For this review, take the finished solid that the model builds, in its own axes (mm). Give positions to 0.01 mm unless a question says otherwise; leave off trailing zeros. Write each loop counter-clockwise with the first axis right and the second up, starting at its lowest first coordinate (ties: lowest second). Pieces come first, ordered by that corner, then holes.
Q1. We need section A-A (y = 63.5). Write out the cut boundary in (x, z).
Q2. For line 1 (Y direction, x = 111.5, z = 4.75); line 2 (Y direction, x = 125, z = 1.2); line 3 (X direction, y = 19.5, z = 1.9), list the stretches that pass through material, from the lowest coordinate up.
Q3. Insertion check: P1, Ø1.8, axis at x = 105.72, y = -7.19, coming from the -Z side; P2, Ø3.5, axis at x = 125.72, y = 83.81, coming from the +Z side. Each pin has a flat end and moves straight along its axis. Give the tip position at first contact, or say it passes through.
Q4. We need section C-C (z = 3.15). Give the number of separate pieces and of enclosed holes in the cut face, then the cut area to 3 significant figures.
Q5. We need section B-B (x = 92.5). Write out the cut boundary in (y, z).
Q6. We need section D-D (x = 99.5). Write out the cut boundary in (y, z), then the cut area to 3 significant figures.
Autodesk Fusion 360 part; units mm, degrees
sketch "Schizzo5" plane through (0, 0, 0) normal (0, 0, 1) x (1, 0, 0)
  line L0 (80.7173, 86.3147) -> (80.7173, -9.6853)
  circle A0 centre (85.7173, -7.1853) radius 1.5
  circle A1 centre (105.7173, 38.3147) radius 25 construction
  arc A2 (125.5163, 58.1137) -> (105.7173, 66.3147) centre (105.7173, 38.3147) ccw
  circle A3 centre (121.787, 57.4658) radius 3
  circle A4 centre (89.6476, 57.4658) radius 3
  arc A5 (105.7173, 66.3147) -> (85.9183, 58.1137) centre (105.7173, 38.3147) ccw
  circle A6 centre (125.7173, 83.8147) radius 3
  arc A7 (105.7173, 10.3147) -> (125.5163, 18.5157) centre (105.7173, 38.3147) ccw
  line L1 (80.7173, 38.3147) -> (130.7173, 38.3147) construction
  circle A8 centre (105.7173, 83.8147) radius 1.5
  circle A9 centre (85.7173, 83.8147) radius 3
  line L2 (105.7173, 38.3147) -> (121.787, 19.1636) construction
  arc A10 (105.7173, 66.3147) -> (85.9183, 58.1137) centre (105.7173, 38.3147) ccw
  circle A11 centre (85.7173, 83.8147) radius 1.5
  line L3 (130.7173, 86.3147) -> (80.7173, 86.3147)
  arc A12 (125.5163, 58.1137) -> (105.7173, 66.3147) centre (105.7173, 38.3147) ccw
  circle A13 centre (125.7173, 83.8147) radius 1.5
  line L4 (105.7173, 38.3147) -> (89.6274, 54.4047) construction
  circle A14 centre (105.7173, 83.8147) radius 3
  arc A15 (105.7173, 10.3147) -> (125.5163, 18.5157) centre (105.7173, 38.3147) ccw
  line L5 (105.7173, 38.3147) -> (105.7173, 13.3147) construction
  circle A16 centre (105.7173, 38.3147) radius 4.1
  circle A17 centre (105.7173, -7.1853) radius 1.5
  circle A18 centre (89.6476, 19.1636) radius 3
  line L6 (130.7173, -9.6853) -> (130.7173, 86.3147)
  arc A19 (85.9183, 18.5157) -> (105.7173, 10.3147) centre (105.7173, 38.3147) ccw
  line L7 (85.7173, 86.3147) -> (85.7173, -9.6853) construction
  arc A20 (105.7173, 13.3147) -> (121.787, 19.1636) centre (105.7173, 38.3147) ccw
  circle A21 centre (121.787, 19.1636) radius 3
  circle A22 centre (85.7173, -7.1853) radius 3
  circle A23 centre (105.7173, -7.1853) radius 3
  circle A24 centre (125.7173, -7.1853) radius 1.5
  line L8 (105.7173, 38.3147) -> (123.668, 56.2654) construction
  line L9 (80.7173, -9.6853) -> (130.7173, -9.6853)
  circle A25 centre (125.7173, -7.1853) radius 3
  line L10 (80.7173, -7.1853) -> (130.7173, -7.1853) construction
  line L11 (105.7173, 38.3147) -> (89.6476, 19.1636) construction
  arc A26 (85.9183, 18.5157) -> (105.7173, 10.3147) centre (105.7173, 38.3147) ccw
  line L12 (105.7173, 86.3147) -> (105.7173, -9.6853) construction
  arc A27 (89.6476, 19.1636) -> (105.7173, 13.3147) centre (105.7173, 38.3147) ccw
  line L13 (105.7173, 38.3147) -> (105.7173, 63.3147) construction
  line L14 (105.7173, 38.3147) -> (105.7173, 63.3147) construction
  line L15 (105.7173, 38.3147) -> (105.7173, 13.3147) construction
  arc A28 (105.7173, 16.3147) -> (121.2737, 22.7584) centre (105.7173, 38.3147) ccw
  arc A29 (90.161, 22.7584) -> (105.7173, 16.3147) centre (105.7173, 38.3147) ccw
  arc A30 (105.7173, 60.3147) -> (90.161, 53.8711) centre (105.7173, 38.3147) ccw
  arc A31 (121.2737, 53.8711) -> (105.7173, 60.3147) centre (105.7173, 38.3147) ccw
  dimension "d219" = 3
  dimension "d220" = 3
  dimension "d221" = 50
  dimension "d222" = 96
  dimension "d223" = 2.5
  dimension "d224" = 20
  dimension "d225" = 3
  dimension "d226" = 6
  dimension "d227" = 3
  dimension "d228" = 6
  dimension "d229" = 8.2
  dimension "d230" = 40
  dimension "d231" = 6
  dimension "d232" = 40
  dimension "d233" = 6
  dimension "d246" = -3
  dimension "d247" = -3
extrude "Estrusione24" add sketch "Schizzo5" along normal blind 5 contours L0 A6 A9 L3 A14 L6 A22 A23 L9 A25
extrude "Estrusione25" add sketch "Schizzo5" along normal blind 1.8 contours A9 L3 | A22 L9 | L3 A14 | A23 L9 | A6 L3 | L9 A25 picked at (85.7547, 85.98) picked at (85.7547, -9.3505) picked at (105.7547, 85.98) picked at (105.7547, -9.3505) picked at (125.7547, 85.98) picked at (125.7547, -9.3505)
equation "d225 = d227"
equation "d226 = d228"
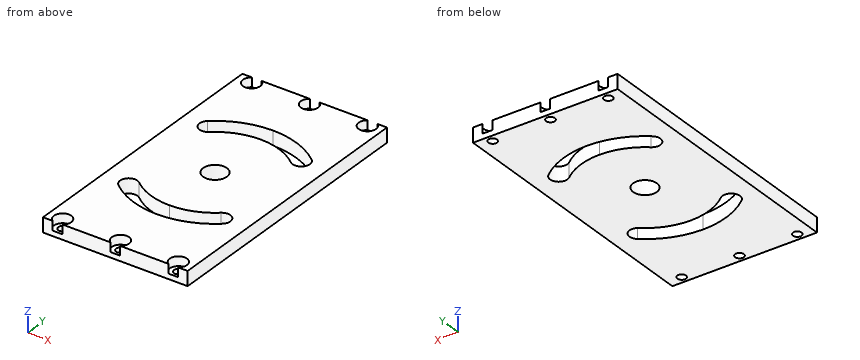
Computed:
1. outline: (80.72, 0) - (93.48, 0) - (93.48, 5) - (80.72, 5) - close; (117.95, 0) - (130.72, 0) - (130.72, 5) - (117.95, 5) - close
2. line 1: y = -9.69 to 10.92, 17.09 to 59.54, 65.71 to 86.31
2. line 2: y = -9.69 to -8.5, -5.87 to 82.5, 85.13 to 86.31
2. line 3: x = 80.72 to 86.67, 94.32 to 117.12, 124.77 to 130.72
3. P1: passes through
3. P2: stops at z = 1.8
4. separate pieces: 1
4. enclosed holes: 3
4. area: 4,110 mm2
5. outline: (-9.69, 0) - (13.63, 0) - (13.63, 5) - (-9.69, 5) - close; (20.73, 0) - (55.9, 0) - (55.9, 5) - (20.73, 5) - close; (63, 0) - (86.31, 0) - (86.31, 5) - (63, 5) - close
6. outline: (-9.69, 0) - (11.01, 0) - (11.01, 5) - (-9.69, 5) - close; (17.21, 0) - (59.42, 0) - (59.42, 5) - (17.21, 5) - close; (65.62, 0) - (86.31, 0) - (86.31, 5) - (65.62, 5) - close
6. area: 418 mm2
